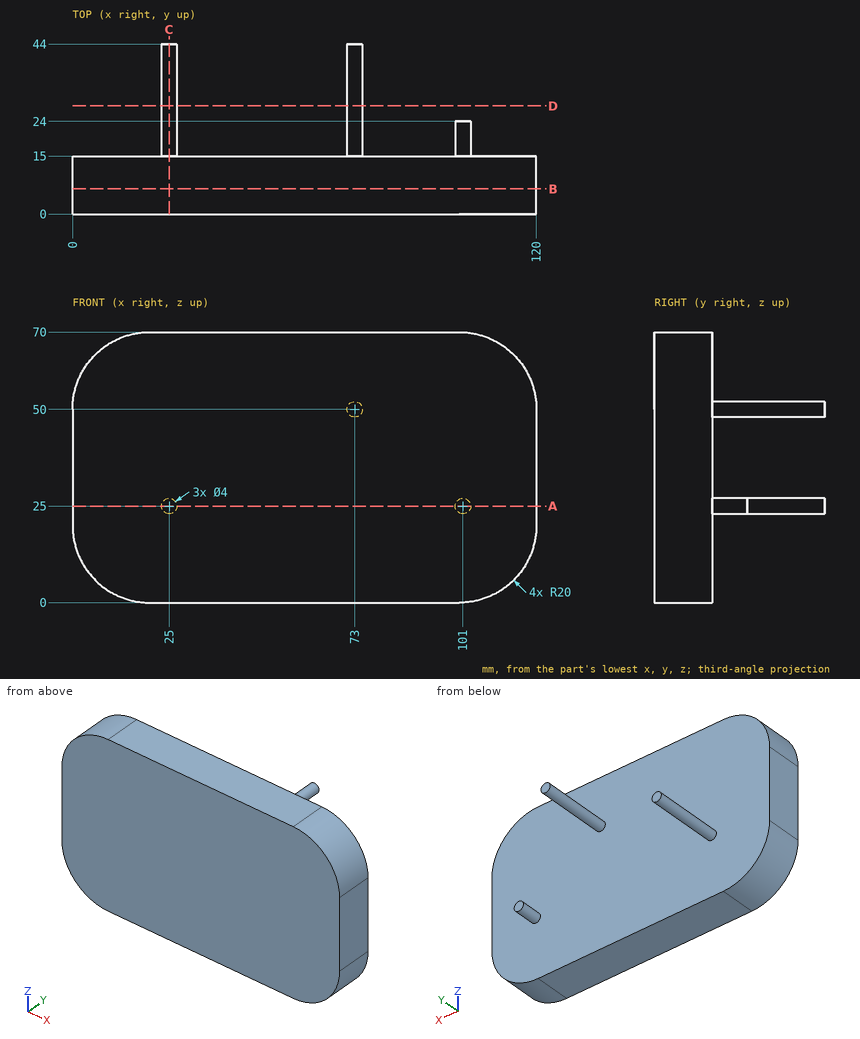
Study the drawing (mm; zero at the part's minimum x, y, z) and answer. Give positions to 0.01 mm unless a question says otherwise; leave off trailing zeros. Write each loop counter-clockwise with the first axis right and the second up, starting at its lowest first coordinate (ties: lowest second). Pieces come first, ordered by that corner, then holes.
(1) The part is cut by section B-B on y = 6.5. Write down the section's boundary in (x, z), plus the area to 3 significant figures.
Final values:
outline: (0, 20) arc R20 ccw to (20, 0) - (100, 0) arc R20 ccw to (120, 20) - (120, 50) arc R20 ccw to (100, 70) - (20, 70) arc R20 ccw to (0, 50) - close
area: 8,060 mm2
(2) The part is cut by section D-D on y = 28. Write down the section's boundary in (x, z), plus the area to 3 significant figures.
Final values:
outline: circle Ø4 at (25, 25); circle Ø4 at (73, 50)
area: 25.1 mm2
(3) The part is cut by section C-C on x = 25. Write down the section's boundary in (y, z).
Final values:
outline: (0, 0) - (15, 0) - (15, 23) - (44, 23) - (44, 27) - (15, 27) - (15, 70) - (0, 70) - close
(4) The part is cut by section A-A on z = 25. Write down the section's boundary in (x, y).
Final values:
outline: (0, 0) - (120, 0) - (120, 15) - (103, 15) - (103, 24) - (99, 24) - (99, 15) - (27, 15) - (27, 44) - (23, 44) - (23, 15) - (0, 15) - close
(5) Flat-ended cylindrical pins translate along their axes: pin 1 Ø3 at (y, z) = (27.5, 53) entering from -X; pin 2 Ø8 at (y, z) = (27, 53) entering from -X; pin 3 Ø1.2 at (x, z) = (101.5, 25) entering from +Y. Find the tip coordinate at first contact, or state that the pin passes through.
Final values:
pin 1: stops at x = 71.68
pin 2: stops at x = 71
pin 3: stops at y = 24
(6) Straight lines are drawn through the part: line 1 (Y direction, x = 100, z = 21.5); line 2 (X direction, y = 5.5, z = 13) (3 decimals); line 3 (X direction, y = 24, z = 51.5). For each, find the intervals that lie inside material, in ascending order.
Final values:
line 1: y = 0 to 15
line 2: x = 1.265 to 118.735
line 3: x = 71.68 to 74.32
